from build123d import *

# Parameters (mm, degrees)
BOSS_EXTRUDE1_DEPTH = 3
BOSS_EXTRUDE2_DEPTH = 3
CUT_EXTRUDE1_DEPTH  = 4
SKETCH5_R           = 1.5
CUT_EXTRUDE2_DEPTH  = 10
SKETCH7_R           = 4
CUT_EXTRUDE3_DEPTH  = 6
SKETCH8_R           = 1.5
CUT_EXTRUDE4_DEPTH  = 4
CUT_EXTRUDE5_DEPTH  = 10
CUT_EXTRUDE6_DEPTH  = 4


with BuildPart() as part:
    # Sketch2 → Boss-Extrude1 (new body)
    with BuildSketch(Plane.XY):
        Polygon((-110, 49.75), (3, 49.75), (3, 80), (-157, 80), (-157, -80), (3, -80), (3, -49.75), (-110, -49.75), align=None)
    extrude(amount=BOSS_EXTRUDE1_DEPTH)

    # Sketch3 → Boss-Extrude2 (add)
    with BuildSketch(Plane.XY.offset(3)):
        Polygon((-77.5, 38), (-41.5, 38), (-29.75, 49.75), (-84.283865663, 49.75), align=None)
        Polygon((-29.75, -49.75), (-84.283865663, -49.75), (-77.5, -38), (-41.5, -38), align=None)
    extrude(amount=-BOSS_EXTRUDE2_DEPTH)

    # Sketch4 → Cut-Extrude1 (cut, through all)
    with BuildSketch(Plane.XY.offset(3)):
        Polygon((-17.886751346, -49.75), (-15, -54.75), (3, -54.75), (3, -49.75), align=None)
        Polygon((-17.886751346, 49.75), (-15, 54.75), (3, 54.75), (3, 49.75), align=None)
    extrude(amount=-CUT_EXTRUDE1_DEPTH, mode=Mode.SUBTRACT)

    # Sketch5 → Cut-Extrude2 (cut)
    with BuildSketch(Plane.XY.offset(3)):
        with Locations((-73, -42.65)):
            Circle(SKETCH5_R)
        with Locations((-46, -42.65)):
            Circle(SKETCH5_R)
        with Locations((-46, -53.35)):
            Circle(SKETCH5_R)
        with Locations((-73, -53.35)):
            Circle(SKETCH5_R)
        with Locations((-46, 42.65)):
            Circle(SKETCH5_R)
        with Locations((-73, 42.65)):
            Circle(SKETCH5_R)
        with Locations((-73, 53.35)):
            Circle(SKETCH5_R)
        with Locations((-46, 53.35)):
            Circle(SKETCH5_R)
    extrude(amount=-CUT_EXTRUDE2_DEPTH, mode=Mode.SUBTRACT)

    # Sketch7 → Cut-Extrude3 (cut)
    with BuildSketch(Plane(origin=(0, 0, 0), x_dir=(-1, 0, 0), z_dir=(0, 0, -1))):
        with Locations((28.811352149, -59.5)):
            Circle(SKETCH7_R)
        with Locations((28.811352149, 59.5)):
            Circle(SKETCH7_R)
    extrude(amount=-CUT_EXTRUDE3_DEPTH, mode=Mode.SUBTRACT)

    # Sketch8 → Cut-Extrude4 (cut)
    with BuildSketch(Plane.XY.offset(3)):
        with Locations((-17.811352149, 59.1)):
            Circle(SKETCH8_R)
        with Locations((-17.811352149, 71.1)):
            Circle(SKETCH8_R)
        with Locations((-42.811352149, 63.1)):
            Circle(SKETCH8_R)
        with Locations((-42.811352149, 71.1)):
            Circle(SKETCH8_R)
        with Locations((-42.811352149, -71.1)):
            Circle(SKETCH8_R)
        with Locations((-42.811352149, -63.1)):
            Circle(SKETCH8_R)
        with Locations((-17.811352149, -59.1)):
            Circle(SKETCH8_R)
        with Locations((-17.811352149, -71.1)):
            Circle(SKETCH8_R)
    extrude(amount=-CUT_EXTRUDE4_DEPTH, mode=Mode.SUBTRACT)

    # Sketch9 → Cut-Extrude5 (cut)
    with BuildSketch(Plane(origin=(0, 0, 0), x_dir=(-1, 0, 0), z_dir=(0, 0, -1))):
        with BuildLine():
            Line((32.811352149, -55.5), (28.811352149, -55.5))
            ThreePointArc((28.811352149, -55.5), (31.639779274, -56.671572875), (32.811352149, -59.5))
            Line((32.811352149, -59.5), (32.811352149, -55.5))
        make_face()
        with BuildLine():
            Line((24.811352149, -55.5), (24.811352149, -59.5))
            ThreePointArc((24.811352149, -59.5), (25.982925025, -56.671572875), (28.811352149, -55.5))
            Line((28.811352149, -55.5), (24.811352149, -55.5))
        make_face()
        with BuildLine():
            ThreePointArc((28.811352149, 55.5), (25.982925025, 56.671572875), (24.811352149, 59.5))
            Line((24.811352149, 59.5), (24.811352149, 55.5))
            Line((24.811352149, 55.5), (28.811352149, 55.5))
        make_face()
        with BuildLine():
            Line((32.811352149, 55.5), (32.811352149, 59.5))
            ThreePointArc((32.811352149, 59.5), (31.639779274, 56.671572875), (28.811352149, 55.5))
            Line((28.811352149, 55.5), (32.811352149, 55.5))
        make_face()
    extrude(amount=-CUT_EXTRUDE5_DEPTH, mode=Mode.SUBTRACT)

    # Sketch10 → Cut-Extrude6 (cut, through all)
    with BuildSketch(Plane(origin=(0, 0, 0), x_dir=(-1, 0, 0), z_dir=(0, 0, -1))):
        with BuildLine():
            Line((71.5, -52.6), (71.5, -53.35))
            ThreePointArc((71.5, -53.35), (73, -51.85), (74.5, -53.35))
            Line((74.5, -53.35), (74.5, -52.6))
            ThreePointArc((74.5, -52.6), (73, -51.1), (71.5, -52.6))
        make_face()
        with BuildLine():
            Line((71.5, -53.35), (71.5, -54.1))
            ThreePointArc((71.5, -54.1), (73, -55.6), (74.5, -54.1))
            Line((74.5, -54.1), (74.5, -53.35))
            ThreePointArc((74.5, -53.35), (73, -54.85), (71.5, -53.35))
        make_face()
        with BuildLine():
            Line((74.5, -43.4), (74.5, -42.65))
            ThreePointArc((74.5, -42.65), (73, -44.15), (71.5, -42.65))
            Line((71.5, -42.65), (71.5, -43.4))
            ThreePointArc((71.5, -43.4), (73, -44.9), (74.5, -43.4))
        make_face()
        with BuildLine():
            Line((74.5, -42.65), (74.5, -41.9))
            ThreePointArc((74.5, -41.9), (73, -40.4), (71.5, -41.9))
            Line((71.5, -41.9), (71.5, -42.65))
            ThreePointArc((71.5, -42.65), (73, -41.15), (74.5, -42.65))
        make_face()
        with BuildLine():
            Line((47.5, -42.65), (47.5, -41.9))
            ThreePointArc((47.5, -41.9), (46, -40.4), (44.5, -41.9))
            Line((44.5, -41.9), (44.5, -42.65))
            ThreePointArc((44.5, -42.65), (46, -41.15), (47.5, -42.65))
        make_face()
        with BuildLine():
            Line((47.5, -43.4), (47.5, -42.65))
            ThreePointArc((47.5, -42.65), (46, -44.15), (44.5, -42.65))
            Line((44.5, -42.65), (44.5, -43.4))
            ThreePointArc((44.5, -43.4), (46, -44.9), (47.5, -43.4))
        make_face()
        with BuildLine():
            Line((44.5, -52.6), (44.5, -53.35))
            ThreePointArc((44.5, -53.35), (46, -51.85), (47.5, -53.35))
            Line((47.5, -53.35), (47.5, -52.6))
            ThreePointArc((47.5, -52.6), (46, -51.1), (44.5, -52.6))
        make_face()
        with BuildLine():
            Line((44.5, -53.35), (44.5, -54.1))
            ThreePointArc((44.5, -54.1), (46, -55.6), (47.5, -54.1))
            Line((47.5, -54.1), (47.5, -53.35))
            ThreePointArc((47.5, -53.35), (46, -54.85), (44.5, -53.35))
        make_face()
    extrude(amount=-CUT_EXTRUDE6_DEPTH, mode=Mode.SUBTRACT)


solid = part.part
Source: CAD feature listing. Evaluate the final solid. Frame: model axes, mm. A direction names the side the tool comes from. Coordinates: 2 decimals unless noted, no trailing zeros. Loops run counter-clockwise (first coordinate to the right, second up) from the corner with the lowest first, then second, coordinate; pieces in that order, holes last. Notation, with made-up numbers: (49, 29.25) - (101, 29.25) arc R36 cw to (101, 66.25) - close; hole circle Ø7 at (-39, 51.5). An arc over 180 degrees is marked (long way). One line per item, written item: value. Start each with the question number.
1. Section B-B (x = -80). Return the cut outline in (y, z).
2. Section A-A (z = 1.75). State how many separate pieces and enclosed holes the cut face has, and give its area (3 significant figures).
3. Ray query, L1, parallel to X at y = 71.1, z = 2.1; L2, parallel to Y at x = -73, z = 2.1; L3, parallel to Y at x = -4.5, z = 1.6. Return the intervals inside material, ascending.
4. Mould query, pull axis Y, two halves, no side actions, for faces 4 (the flat face through (-114, 1, 3)), 5 (the flat face through (-35.7, -43.8, 1.5)). Classes: pulls with the +Y half, pulls with the -Y half, needs draft (parallel to the pull), parting line crosses it, or undercut.
5. Contact query for flat-ended pins moving along their axis: P1, Ø1.2, axis at y = -42.5, z = 1, coming from the +X side; P2, Ø2.5, axis at x = -46, y = 53.35, coming from the -Z side; P3, Ø1.5, axis at y = -10, z = 1, coming from the +X side; P4, Ø1.2, axis at y = -53.5, z = 1.5, coming from the +X side. Output: stop coordinate, or through.
6. Section C-C (y = 29). Return the cut outline in (x, z).
7. Set-up query: faces 1 (the cylindrical face through (-28.7, -63.5, 1.5)), 2 (the flat face through (-35.7, 43.8, 1.5)), 3 (the flat face through (-114, 1, 0)). Return all of +Z, -Z, +X, -X, +Y, -Y with unobstructed straight access to the full face (end or side cutting, diameter ignored); none if empty.
Verdict:
1. outline: (-80, 0) - (-42.33, 0) - (-42.33, 3) - (-80, 3) - close; (42.33, 0) - (80, 0) - (80, 3) - (42.33, 3) - close
2. separate pieces: 1
2. enclosed holes: 18
2. area: 15,000 mm2
3. L1: x = -157 to -44.31, -41.31 to -19.31, -16.31 to 3
3. L2: y = -80 to -55.6, -51.1 to -44.9, -40.4 to -38, 38 to 41.15, 44.15 to 51.85, 54.85 to 80
3. L3: y = -80 to -54.75, 54.75 to 80
4. face 4: needs draft
4. face 5: undercut
5. P1: stops at x = -36.4
5. P2: passes through
5. P3: stops at x = -110
5. P4: stops at x = -15.38
6. outline: (-157, 0) - (-110, 0) - (-110, 3) - (-157, 3) - close
7. face 1: +Z, -Z
7. face 2: +Z, -Z, +X
7. face 3: -Z, +X, -X, +Y, -Y
